Here's how the part is built. I have some questions about the finished solid (model axes, mm). A direction names the side the tool comes from. Coordinates: 2 decimals unless noted, no trailing zeros. Order: outer loops, then holes, each group sorted by start corner. A loop starts at its lowest first (then second) coordinate and runs counter-clockwise, first axis right, second up. Notation, with made-up numbers: (11, 56.25) - (59, 56.25) arc R28 ccw to (59, 82.25) - close; hole circle Ø2 at (49.5, 25). An arc over 180 degrees is marked (long way). Use one line per item in the form item = value. Start each with the question number.
from build123d import *

# Parameters (mm, degrees)
F1_DEPTH  = 3.15
F2_R      = 3.14
F5_DEPTH  = 1.54
F4_R      = 1.5
F4_R_2    = 1.75
F6_DEPTH  = 12.5
F8_DEPTH  = 2.5
F9_W      = 0.62
F9_H      = 0.62
F10_DEPTH = 1.88
F11_W     = 0.62
F11_H     = 0.62
F12_DEPTH = 1.36
F13_W     = 0.62
F13_H     = 0.62
F14_DEPTH = 7.85
F15_R     = 0.5
F16_W     = 3.85
F16_H     = 5
F17_DEPTH = 1.4


with BuildPart() as f1:
    # F0 (on Top) → F1 (new body, symmetric)
    with BuildSketch(Plane.XY):
        Polygon((0, 2.965), (0, 0), (0, -2.965), (-8.13, -2.965), (-8.13, -7.005), (0.41, -7.005), (0.41, -12.965), (3.13, -12.965), (3.13, 0), (3.13, 12.965), (0.41, 12.965), (0.41, 7.005), (-8.13, 7.005), (-8.13, 2.965), align=None)
    extrude(amount=F1_DEPTH, both=True)

    # F2
    f2_edges = [f1.edges().sort_by_distance(p)[0] for p in [
        (1.77, 12.965, 3.15),
        (1.77, 12.965, -3.15),
        (1.77, -12.965, 3.15),
        (1.77, -12.965, -3.15),
    ]]
    fillet(f2_edges, radius=F2_R)

    # F3 (on face) → F5 (join)
    with BuildSketch(Plane.YZ.offset(3.13)):
        with BuildLine():
            Line((-9.9, -3.67), (-9.9, -18.73))
            Line((-9.9, -18.73), (9.9, -18.73))
            Line((9.9, -18.73), (9.9, -3.67))
            ThreePointArc((9.9, -3.67), (6.23, 0), (9.9, 3.67))
            Line((9.9, 3.67), (-9.9, 3.67))
            ThreePointArc((-9.9, 3.67), (-7.304918, 2.595082), (-6.23, 0))
            ThreePointArc((-6.23, 0), (-7.304918, -2.595082), (-9.9, -3.67))
        make_face()
        with BuildLine():
            ThreePointArc((-9.9, 3.67), (-13.57, 0), (-9.9, -3.67))
            ThreePointArc((-9.9, -3.67), (-7.304918, -2.595082), (-6.23, 0))
            ThreePointArc((-6.23, 0), (-7.304918, 2.595082), (-9.9, 3.67))
        make_face()
        with BuildLine():
            ThreePointArc((9.9, 3.67), (6.23, 0), (9.9, -3.67))
            ThreePointArc((9.9, -3.67), (12.495082, -2.595082), (13.57, 0))
            ThreePointArc((13.57, 0), (12.495082, 2.595082), (9.9, 3.67))
        make_face()
    extrude(amount=F5_DEPTH)

    # F4 (on face) → F6 (cut, symmetric)
    with BuildSketch(Plane.YZ.offset(3.13)):
        with Locations((-10.4, 0)):
            Circle(F4_R)
        with Locations((10.4, 0)):
            Circle(F4_R)
        with Locations((-7.75, -7.68)):
            Circle(F4_R_2)
        with Locations((7.75, -7.68)):
            Circle(F4_R_2)
    extrude(amount=F6_DEPTH, both=True, mode=Mode.SUBTRACT)

    # F7 (on face) → F8 (join)
    with BuildSketch(Plane.YZ.offset(4.67)):
        with BuildLine():
            ThreePointArc((1.291667, -16.098165), (1.174071, -15.814263), (0.890169, -15.696667))
            Line((0.890169, -15.696667), (-0.890169, -15.696667))
            ThreePointArc((-0.890169, -15.696667), (-1.174071, -15.814263), (-1.291667, -16.098165))
            Line((-1.291667, -16.098165), (-1.291667, -17.878502))
            ThreePointArc((-1.291667, -17.878502), (-1.174071, -18.162404), (-0.890169, -18.28))
            Line((-0.890169, -18.28), (0.890169, -18.28))
            ThreePointArc((0.890169, -18.28), (1.174071, -18.162404), (1.291667, -17.878502))
            Line((1.291667, -17.878502), (1.291667, -16.098165))
        make_face()
        with BuildLine():
            ThreePointArc((1.693165, -15.696667), (1.409263, -15.814263), (1.291667, -16.098165))
            Line((1.291667, -16.098165), (1.291667, -17.878502))
            ThreePointArc((1.291667, -17.878502), (1.409263, -18.162404), (1.693165, -18.28))
            Line((1.693165, -18.28), (3.473502, -18.28))
            ThreePointArc((3.473502, -18.28), (3.757404, -18.162404), (3.875, -17.878502))
            Line((3.875, -17.878502), (3.875, -16.098165))
            ThreePointArc((3.875, -16.098165), (3.757404, -15.814263), (3.473502, -15.696667))
            Line((3.473502, -15.696667), (1.693165, -15.696667))
        make_face()
        with BuildLine():
            Line((-1.291667, -17.878502), (-1.291667, -16.098165))
            ThreePointArc((-1.291667, -16.098165), (-1.409263, -15.814263), (-1.693165, -15.696667))
            Line((-1.693165, -15.696667), (-3.473502, -15.696667))
            ThreePointArc((-3.473502, -15.696667), (-3.757404, -15.814263), (-3.875, -16.098165))
            Line((-3.875, -16.098165), (-3.875, -17.878502))
            ThreePointArc((-3.875, -17.878502), (-3.757404, -18.162404), (-3.473502, -18.28))
            Line((-3.473502, -18.28), (-1.693165, -18.28))
            ThreePointArc((-1.693165, -18.28), (-1.409263, -18.162404), (-1.291667, -17.878502))
        make_face()
    extrude(amount=F8_DEPTH)

    # F9 (on face) → F10 (join)
    with BuildSketch(Plane.YZ.offset(7.17)):
        with Locations((0, -16.988333)):
            Rectangle(F9_W, F9_H)
        with Locations((2.583333, -16.988333)):
            Rectangle(F9_W, F9_H)
        with Locations((-2.583333, -16.988333)):
            Rectangle(F9_W, F9_H)
    extrude(amount=F10_DEPTH)

    # F11 (on face) → F12 (join)
    with BuildSketch(Plane.YZ.offset(3.13)):
        with Locations((-2.583333, -16.988333)):
            Rectangle(F11_W, F11_H)
        with Locations((0, -16.988333)):
            Rectangle(F11_W, F11_H)
        with Locations((2.583333, -16.988333)):
            Rectangle(F11_W, F11_H)
    extrude(amount=-F12_DEPTH)

    # F13 (on face) → F14 (join)
    with BuildSketch(Plane(origin=(0, 0, -17.298333), x_dir=(1, 0, 0), z_dir=(0, 0, -1))):
        with Locations((8.74, 2.583333)):
            Rectangle(F13_W, F13_H)
        with Locations((8.74, 0)):
            Rectangle(F13_W, F13_H)
        with Locations((8.74, -2.583333)):
            Rectangle(F13_W, F13_H)
    extrude(amount=-F14_DEPTH)

    # F15
    f15_edges = [f1.edges().sort_by_distance(p)[0] for p in [
        (9.05, 2.583333, -17.298333),
        (9.05, 0, -17.298333),
        (9.05, -2.583333, -17.298333),
        (8.43, 2.583333, -16.678333),
        (8.43, 0, -16.678333),
        (8.43, -2.583333, -16.678333),
    ]]
    fillet(f15_edges, radius=F15_R)

    # F16 (on face) → F17 (join)
    with BuildSketch(Plane.YZ.offset(4.67)):
        with Locations((-1.275, -7.68)):
            Rectangle(F16_W, F16_H)
    extrude(amount=F17_DEPTH)


solid = f1.part
1) Suppose I cut it at B-B, the plane z = -7.68. List the corners of the cut face in (x, y) for me, then the cut area to 3 significant figures.
2) Suppose I cut it at A-A, the plane y = 7.75. List the corners of the cut face in (x, z) for me, then the cut area to 3 significant figures.
3) Suppose I cut it at D-D, the plane x = 4. List the corners of the cut face in (y, z) for me, then the cut area to 3 significant figures.
4) If we mould it in two halves opening along Y, with no side actions, what happens to faces 4 (the flat face through (6, 3.875, -17)), 5 (the flat face through (7.17, 0, -16)), 6 (the flat face through (8.7, -0.31, -14.3)), 7 (the flat face through (1, 0, -3.15))? For each: pulls with the +Y half, pulls with the -Y half, needs draft (parallel to the pull), parting line crosses it, or undercut.
5) For pin 1 (10 mm diameter, centred on x = -5, y = 8.5, fed in from +Z); pin 2 (0.5 mm diameter, centred on x = 2.5, y = 2.5, fed in from -Z); pin 3 (7 mm diameter, centred on x = -5.5, z = -1.5, fed in from -Y) (3 decimals), each with a flat end and sliding along its axis, tell me the tip position at first contact or that it passes through.
6) Which directions (+Z, -Z, +X, -X, +Y, -Y) give clear straight access to the entire face, cutting with the end or side of a thin tool? Please do faces 1 (the flat face through (0.41, 8.7, 0)), 2 (the flat face through (6, 0, -18.28)), 3 (the flat face through (8.7, -2.893, -14.3)).
7) I need wall thicknesses on probe 1 along Z at (x, y) = (4.05, 7.75); probe 2 along Z at (x, y) = (1.7, 10.4); probe 3 along Y at (x, z) = (-6.75, 2.5) (3 decimals). Which ranges of each line are inside material? Lowest first, please. Write a range as [from, to].
8) Suppose I cut it at C-C, the plane x = -6.25. List the corners of the cut face in (y, z) for me (3 decimals).
From the geometry:
q1.outline = (3.13, -9.9) - (4.67, -9.9) - (4.67, -9.5) - (3.13, -9.5) - close; (3.13, -6) - (4.67, -6) - (4.67, -3.2) - (6.07, -3.2) - (6.07, 0.65) - (4.67, 0.65) - (4.67, 6) - (3.13, 6) - close; (3.13, 9.5) - (4.67, 9.5) - (4.67, 9.9) - (3.13, 9.9) - close
q1.area = 25.1 mm2
q2.outline = (0.41, -3.15) - (3.13, -3.15) - (3.13, -5.93) - (4.67, -5.93) - (4.67, 3.67) - (3.13, 3.67) - (3.13, 3.15) - (0.41, 3.15) - close; (3.13, -18.73) - (4.67, -18.73) - (4.67, -9.43) - (3.13, -9.43) - close
q2.area = 46.2 mm2
q3.outline = (-9.9, -18.73) - (9.9, -18.73) - (9.9, -3.67) arc R3.67 ccw to (9.9, 3.67) - (-9.9, 3.67) arc R3.67 ccw to (-9.9, -3.67) - close; hole circle Ø3 at (-10.4, 0); hole circle Ø3.5 at (-7.75, -7.68); hole circle Ø3.5 at (7.75, -7.68); hole circle Ø3 at (10.4, 0)
q3.area = 452 mm2
q4.face_4 = pulls with the +Y half
q4.face_5 = undercut
q4.face_6 = undercut
q4.face_7 = needs draft
q5.pin_1 = 3.15
q5.pin_2 = -17.3
q5.pin_3 = -7.005
q6.face_1 = +Z, -Z, -X, +Y
q6.face_2 = -Z, +X, +Y, -Y
q6.face_3 = +Z, -Z, +X, -Y
q7.probe_1 = [-18.73, -9.43], [-5.93, 3.67]
q7.probe_2 = [-3.1, -1.5], [1.5, 3.1]
q7.probe_3 = [-7.005, -2.965], [2.965, 7.005]
q8.outline = (-7.005, -3.15) - (-2.965, -3.15) - (-2.965, 3.15) - (-7.005, 3.15) - close; (2.965, -3.15) - (7.005, -3.15) - (7.005, 3.15) - (2.965, 3.15) - close
